```python
from build123d import *

# Parameters (mm, degrees)
SKETCH4_R           = 54
BOSS_EXTRUDE1_DEPTH = 4
FILLET1_R           = 6
SKETCH9_R           = 1.75
CUT_EXTRUDE2_DEPTH  = 50
SKETCH7_R           = 1.75
CUT_EXTRUDE3_DEPTH  = 50


with BuildPart() as part:
    # Sketch2 → Revolve2 (revolve)
    with BuildSketch(Plane.XY, mode=Mode.PRIVATE) as revolve2_sk:
        Polygon((0, 0), (42, 0), (42, 24), (11.5, 24), align=None)
    revolve(revolve2_sk.sketch.rotate(Axis((42, 0, 0), (0, 1, 0)), 270), axis=Axis((42, 0, 0), (0, 1, 0)))

    # Sketch4 → Boss-Extrude1 (add)
    with BuildSketch(Plane.XZ):
        with Locations(Location((42, 0, 0), (0, 0, 270))):
            Circle(SKETCH4_R)
    extrude(amount=BOSS_EXTRUDE1_DEPTH)

    # Fillet1
    fillet1_edges = [part.edges().sort_by_distance(p)[0] for p in [
        (42, 0, 42),
    ]]
    fillet(fillet1_edges, radius=FILLET1_R)

    # Sketch9 → Cut-Extrude2 (cut)
    with BuildSketch(Plane(origin=(0, 24, 0), x_dir=(1, 0, 0), z_dir=(0, 1, 0))):
        with Locations(Location((47.059526539, 26.521711694, 0), (0, 0, 270))):
            Circle(SKETCH9_R)
        with Locations(Location((62.43871281, -17.642534361, 0), (0, 0, 270))):
            Circle(SKETCH9_R)
        with Locations(Location((16.501760651, -8.879177334, 0), (0, 0, 270))):
            Circle(SKETCH9_R)
    extrude(amount=-CUT_EXTRUDE2_DEPTH, mode=Mode.SUBTRACT)

    # Sketch7 → Cut-Extrude3 (cut)
    with BuildSketch(Plane(origin=(0, 0, 0), x_dir=(1, 0, 0), z_dir=(0, 1, 0))):
        with Locations(Location((42.246934907, -49.999390228, 0), (0, 0, 270))):
            Circle(SKETCH7_R)
        with Locations(Location((-1.177274657, -25.213547017, 0), (0, 0, 270))):
            Circle(SKETCH7_R)
        with Locations(Location((-1.424209565, 24.785843211, 0), (0, 0, 270))):
            Circle(SKETCH7_R)
        with Locations(Location((41.753065093, 49.999390228, 0), (0, 0, 270))):
            Circle(SKETCH7_R)
        with Locations(Location((85.177274657, 25.213547017, 0), (0, 0, 270))):
            Circle(SKETCH7_R)
        with Locations(Location((85.424209565, -24.785843211, 0), (0, 0, 270))):
            Circle(SKETCH7_R)
    extrude(amount=-CUT_EXTRUDE3_DEPTH, mode=Mode.SUBTRACT)


solid = part.part
```
Geometry: final body of the model. Coordinates: model frame, mm. A direction names the side the tool comes from. Round coordinates to 2 decimals unless told otherwise and drop trailing zeros. Order: outer loops, then holes, each group sorted by start corner. A loop starts at its lowest first (then second) coordinate and runs counter-clockwise, first axis right, second up. Notation, with made-up numbers: (80, 19) -> (122, 19) arc R16 cw to (122, 45) -> close; hole circle Ø6 at (-28.5, 8). An arc over 180 degrees is marked (long way). Use one line per item in the form item = value. Start each with the question number.
1. Pin query (flat end, axial travel): pin 1 Ø4 at (x, z) = (85.42, 24.79) entering from +Y; pin 2 Ø10 at (x, y) = (49, 9) entering from +Z; pin 3 Ø4 at (y, z) = (9, -7) entering from -X. Return the tip coordinate at first contact, or that it passes through.
2. Line query: probe 1 along Y at (x, z) = (78.5, -29); probe 2 along Z at (x, y) = (48, 3.25); probe 3 along Z at (x, y) = (48.5, 16). Output: solid intervals per line, ascending.
3. Cut plane B-B (y = -1.75). Count the separate pieces of the cut face and the enclosed holes in it, then the cut area to 3 significant figures.
4. Cut plane D-D (y = 4.75). Return the cut outline in (x, z), then the cut area to 3 significant figures.
5. Draft query along X for faces 3 (the face through (42, 24, 0)), 4 (the face through (60.73, 10.2, 17.26)), 5 (the face through (-0.241, -1.972, -26.076)), 6 (the face through (72.377, 22.712, 6.746)). Return one class per face: pulls with the +X half, pulls with the -X half, needs draft (parallel to the pull), parting line crosses it, or undercut.
6. Reachability of faces 1 (the face through (86.3, 0, 12.3)), 2 (the face through (40.045, -1.972, -50.379)) from +Z, -Z, +X, -X, +Y, -Y: full face, straight path, thin tool, end or side. Return the list, or none.
7. Cut plane A-A (z = 0). Return the cut outline in (x, y), then the cut area to 3 significant figures.
8. Cut plane C-C (y = 16.25). Return the cut outline in (x, z), then the cut area to 3 significant figures.
Solution:
q1.pin_1 = 0
q1.pin_2 = 39.59
q1.pin_3 = 3.93
q2.probe_1 = -4 to 0
q2.probe_2 = -40 to -28, -25.05 to 40
q2.probe_3 = -33.71 to -27.52, -25.53 to 33.71
q3.separate_pieces = 1
q3.enclosed_holes = 9
q3.area = 9,070 mm^2
q4.outline = circle Ø79.45 at (42, 0); hole circle Ø3.5 at (16.5, 8.88); hole circle Ø3.5 at (47.06, -26.52); hole circle Ø3.5 at (62.44, 17.64)
q4.area = 4,930 mm^2
q5.face_3 = needs draft
q5.face_4 = undercut
q5.face_5 = undercut
q5.face_6 = parting line crosses it
q6.face_1 = +Y
q6.face_2 = +Y, -Y
q7.outline = (-12, -4) -> (96, -4) -> (96, 0) -> (87.78, 0) arc R6 cw to (82.37, 3.41) -> (72.5, 24) -> (11.5, 24) -> (1.63, 3.41) arc R6 cw to (-3.78, 0) -> (-12, 0) -> close
q7.area = 2,180 mm^2
q8.outline = circle Ø68.43 at (42, 0); hole circle Ø3.5 at (16.5, 8.88); hole circle Ø3.5 at (47.06, -26.52); hole circle Ø3.5 at (62.44, 17.64)
q8.area = 3,650 mm^2
